```python
from build123d import *

# Parameters (mm, degrees)
ESQUISSE1_R        = 1.5
ESQUISSE1_R_2      = 2
ESQUISSE1_R_3      = 1.75
ESQUISSE1_W        = 12.5
ESQUISSE1_H        = 24
ESQUISSE1_W_2      = 5
ESQUISSE1_H_2      = 3
BOSS_EXTRU_1_DEPTH = 3
BOSS_EXTRU_2_DEPTH = 4


with BuildPart() as part:
    # Esquisse1 → Boss.-Extru.1 (new body)
    with BuildSketch(Plane.XY):
        with BuildLine():
            Line((-20, 0), (-30, 0))
            ThreePointArc((-30, 0), (-44.494897428, 10.963763172), (-50, 28.284271247))
            Line((-50, 28.284271247), (-50, 80))
            ThreePointArc((-50, 80), (-44.142135624, 94.142135624), (-30, 100))
            Line((-30, 100), (-26.5, 100))
            Line((-26.5, 100), (-26.5, 98.5))
            Line((-26.5, 98.5), (-23.5, 98.5))
            Line((-23.5, 98.5), (-23.5, 100))
            Line((-23.5, 100), (-20, 100))
            ThreePointArc((-20, 100), (-5.857864376, 94.142135624), (0, 80))
            Line((0, 80), (0, 31.5))
            Line((0, 31.5), (-5, 31.5))
            Line((-5, 31.5), (-5, 28.5))
            Line((-5, 28.5), (0, 28.5))
            ThreePointArc((0, 28.5), (-5.442984974, 11.051946592), (-20, 0))
        make_face()
        with Locations((-10, 30)):
            Circle(ESQUISSE1_R, mode=Mode.SUBTRACT)
        with Locations((-25, 30)):
            Circle(ESQUISSE1_R_2, mode=Mode.SUBTRACT)
        with Locations((-15, 50)):
            Circle(ESQUISSE1_R, mode=Mode.SUBTRACT)
        with Locations((-5, 50)):
            Circle(ESQUISSE1_R, mode=Mode.SUBTRACT)
        with Locations((-4.5, 80)):
            Circle(ESQUISSE1_R_3, mode=Mode.SUBTRACT)
        with Locations((-25, 95)):
            Circle(ESQUISSE1_R, mode=Mode.SUBTRACT)
        with Locations((-39.25, 38)):
            Rectangle(ESQUISSE1_W, ESQUISSE1_H, mode=Mode.SUBTRACT)
        with Locations((-17.5, 30)):
            Rectangle(ESQUISSE1_W_2, ESQUISSE1_H_2, mode=Mode.SUBTRACT)
        Polygon((-42, 24.5), (-34, 24.5), (-34, 23.5), (-27, 23.5), (-27, 22.5), (-41, 22.5), (-41, 20.5), (-27, 20.5), (-27, 19), (-35, 19), (-42, 19), align=None, mode=Mode.SUBTRACT)
        Polygon((-34, 51.5), (-34, 52.5), (-27, 52.5), (-27, 53.5), (-41, 53.5), (-41, 55.5), (-27, 55.5), (-27, 57), (-35, 57), (-42, 57), (-42, 51.5), align=None, mode=Mode.SUBTRACT)
    extrude(amount=BOSS_EXTRU_1_DEPTH)

    # Esquisse2 → Boss.-Extru.2 (add)
    with BuildSketch(Plane.ZY.offset(41)):
        Polygon((3, 22.5), (5, 22.5), (5, 23.5), (7, 22.5), (7, 20.5), (3, 20.5), (0, 20.5), (0, 22.5), align=None)
    boss_extru_2 = extrude(amount=-BOSS_EXTRU_2_DEPTH)

    # Sym_trie1: Boss.-Extru.2 across plane
    add(boss_extru_2.mirror(Plane.ZX.offset(38)))


solid = part.part
```
CAD build for the part. Positions are in the model's coordinates, mm. A direction names the side the tool comes from. Round coordinates to 2 decimals unless told otherwise and drop trailing zeros. Order: outer loops, then holes, each group sorted by start corner. A loop starts at its lowest first (then second) coordinate and runs counter-clockwise, first axis right, second up.
Item 1: Pin check, flat tips, straight feed: pin 1 (1.5 mm diameter, centred on x = -31.5, z = 1.5, fed in from +Y); pin 2 (0.9 mm diameter, centred on y = 22, z = 6, fed in from +X); pin 3 (1.5 mm diameter, centred on x = -40.5, z = 1, fed in from -Y). Stop position of each tip, or through.
Item 2: Probe line 1 along Y through (x, z) = (-25, 1.25); line 2 along X through (y, z) = (34, 2.5); line 3 along Y through (x, z) = (-41.5, 1). List the from-to ranges inside material, lowest first.
Item 3: Tool access for faces 1 (the face through (-37, 54, 5)), 2 (the face through (-36, 22.5, 2)), 3 (the face through (-41, 54, 4)), 4 (the face through (-39, 23, 6)), 5 (the face through (-5, 30, 1)): list every direction of +Z, -Z, +X, -X, +Y, -Y with a clear straight run to the whole face (end or side of a thin tool).
Item 4: Saw through at B-B on z = 4. Write the cut outline in (x, y), then the cut area to 3 significant figures.
Item 5: Saw through at D-D on x = -40. Write the cut outline in (y, z), then the cut area to 3 significant figures.
Item 6: Saw through at A-A on y = 30. Write the cut outline in (x, z).
Item 7: Saw through at C-C on x = -25. Write the cut outline in (y, z).
Item 8: Mould opens along X. For faces 6 (the face through (-50, 54, 1)), 7 (the face through (-5.29, 11.27, 1.48)), 8 (the face through (-31, 23.5, 1)) say: pulls with the +X half, pulls with the -X half, needs draft (parallel to the pull), parting line crosses it, or undercut.
Reported:
1. pin 1: stops at y = 99.99
1. pin 2: stops at x = -37
1. pin 3: stops at y = 5.7
2. line 1: y = 0 to 28, 32 to 93.5, 96.5 to 98.5
2. line 2: x = -50 to -45.5, -33 to 0
2. line 3: y = 7.36 to 19, 24.5 to 26, 50 to 51.5, 57 to 96.36
3. face 1: +Z, +X, +Y, -Y
3. face 2: -Z
3. face 3: +Z, -Z
3. face 4: +Z, +X, -X
3. face 5: +Z, -Z, +X
4. outline: (-41, 20.5) - (-37, 20.5) - (-37, 22.5) - (-41, 22.5) - close; (-41, 53.5) - (-37, 53.5) - (-37, 55.5) - (-41, 55.5) - close
4. area: 16.0 mm2
5. outline: (5.92, 0) - (19, 0) - (19, 3) - (5.92, 3) - close; (20.5, 0) - (22.5, 0) - (22.5, 5) - (23.5, 5) - (22.5, 7) - (20.5, 7) - close; (24.5, 0) - (26, 0) - (26, 3) - (24.5, 3) - close; (50, 0) - (51.5, 0) - (51.5, 3) - (50, 3) - close; (52.5, 5) - (53.5, 5) - (53.5, 0) - (55.5, 0) - (55.5, 7) - (53.5, 7) - close; (57, 0) - (97.32, 0) - (97.32, 3) - (57, 3) - close
5. area: 199 mm2
6. outline: (-50, 0) - (-45.5, 0) - (-45.5, 3) - (-50, 3) - close; (-33, 0) - (-27, 0) - (-27, 3) - (-33, 3) - close; (-23, 0) - (-20, 0) - (-20, 3) - (-23, 3) - close; (-15, 0) - (-11.5, 0) - (-11.5, 3) - (-15, 3) - close; (-8.5, 0) - (-5, 0) - (-5, 3) - (-8.5, 3) - close
7. outline: (0, 0) - (28, 0) - (28, 3) - (0, 3) - close; (32, 0) - (93.5, 0) - (93.5, 3) - (32, 3) - close; (96.5, 0) - (98.5, 0) - (98.5, 3) - (96.5, 3) - close
8. face 6: pulls with the -X half
8. face 7: pulls with the +X half
8. face 8: undercut
